```python
from build123d import *

# Parameters (mm, degrees)
SKETCH4_R          = 1.85
CUT_EXTRUDE1_DEPTH = 6
CIRPATTERN1_COUNT  = 10


with BuildPart() as part:
    # Sketch3 (on Front Plane) → Revolve2 (revolve)
    with BuildSketch(Plane.XY, mode=Mode.PRIVATE) as revolve2_sk:
        with BuildLine():
            Line((-117.849137803, -13.05), (-113, -13.05))
            ThreePointArc((-113, -13.05), (-112.292893219, -13.342893219), (-112, -14.05))
            Line((-112, -14.05), (-112, -18.100862197))
            Line((-112, -18.100862197), (-114.05, -20.150862197))
            Line((-114.05, -20.150862197), (-114.05, -29))
            Line((-114.05, -29), (-125, -29))
            Line((-125, -29), (-125, -12))
            ThreePointArc((-125, -12), (-124.707106781, -11.292893219), (-124, -11))
            Line((-124, -11), (-119.899137803, -11))
            Line((-119.899137803, -11), (-117.849137803, -13.05))
        make_face()
    revolve(revolve2_sk.sketch.rotate(Axis((0, 0, 0), (0, 1, 0)), 270), axis=Axis((0, 0, 0), (0, 1, 0)))

    # Sketch4 → Cut-Extrude1 (cut)
    with BuildSketch(Plane.XZ.offset(29)):
        with Locations(Location((0, -119.525, 0), (0, 0, 270))):
            Circle(SKETCH4_R)
    cut_extrude1 = extrude(amount=-CUT_EXTRUDE1_DEPTH, mode=Mode.SUBTRACT)

    # CirPattern1: Cut-Extrude1 ×10 about axis
    cirpattern1_axis = Axis((0, 0, 0), (0, 1, 0))
    for i in range(1, CIRPATTERN1_COUNT):
        add(cut_extrude1.rotate(cirpattern1_axis, i * 360 / CIRPATTERN1_COUNT), mode=Mode.SUBTRACT)


solid = part.part
```
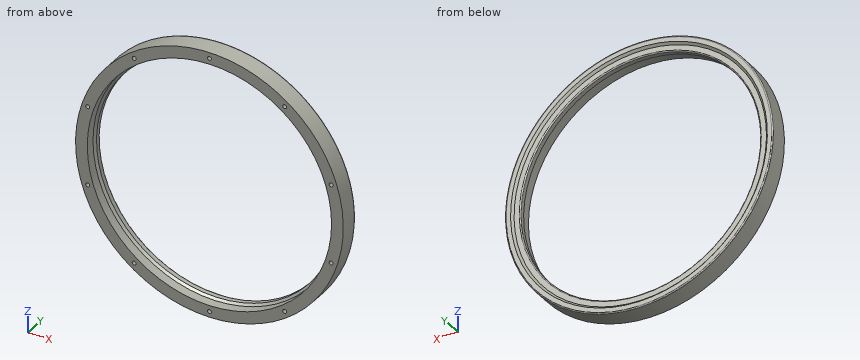
Geometry: final body of the model. Coordinates: model frame, mm. Coordinates: 2 decimals unless noted, no trailing zeros. Loops run counter-clockwise (first coordinate to the right, second up) from the corner with the lowest first, then second, coordinate; pieces in that order, holes last. Notation, with made-up numbers: (-31.5, 68.25) -> (2.5, 68.25) arc R25 cw to (2.5, 90.25) -> close; hole circle Ø3 at (63, -19). An arc over 180 degrees is marked (long way). Use a Markdown table: item, result. Add a question column.
(1) Line query: line 1 along X through (y, z) = (-12, 81); line 2 along X through (y, z) = (-12.25, 64); line 3 along Z through (x, y) = (-57.5, -23.25). Output: solid intervals per line, ascending.
(2) Pin query (flat end, axial travel): pin 1 Ø4 at (y, z) = (-21.5, -33) entering from -X (3 decimals); pin 2 Ø1.8 at (x, z) = (-114, -37.5) entering from -Y; pin 3 Ø2 at (x, y) = (-14.5, -22.5) entering from +Z. Return the tip coordinate at first contact, or that it passes through.
(3) Section query A-A, the plane z = 0. Return loops of the section in (x, y).
Answer:
| question | item | result |
|---|---|---|
| 1 | line 1 | x = -95.21 to -87.04, 87.04 to 95.21 |
| 1 | line 2 | x = -107.37 to -99.91, 99.91 to 107.37 |
| 1 | line 3 | z = -110.99 to -98.49, 98.49 to 110.99 |
| 2 | pin 1 | stops at x = -121.095 |
| 2 | pin 2 | stops at y = -23 |
| 2 | pin 3 | stops at z = 124.27 |
| 3 | outline | (-125, -29) -> (-114.05, -29) -> (-114.05, -20.15) -> (-112, -18.1) -> (-112, -14.05) arc R1 ccw to (-113, -13.05) -> (-117.85, -13.05) -> (-119.9, -11) -> (-124, -11) arc R1 ccw to (-125, -12) -> close; (112, -18.1) -> (114.05, -20.15) -> (114.05, -29) -> (125, -29) -> (125, -12) arc R1 ccw to (124, -11) -> (119.9, -11) -> (117.85, -13.05) -> (113, -13.05) arc R1 ccw to (112, -14.05) -> close |
